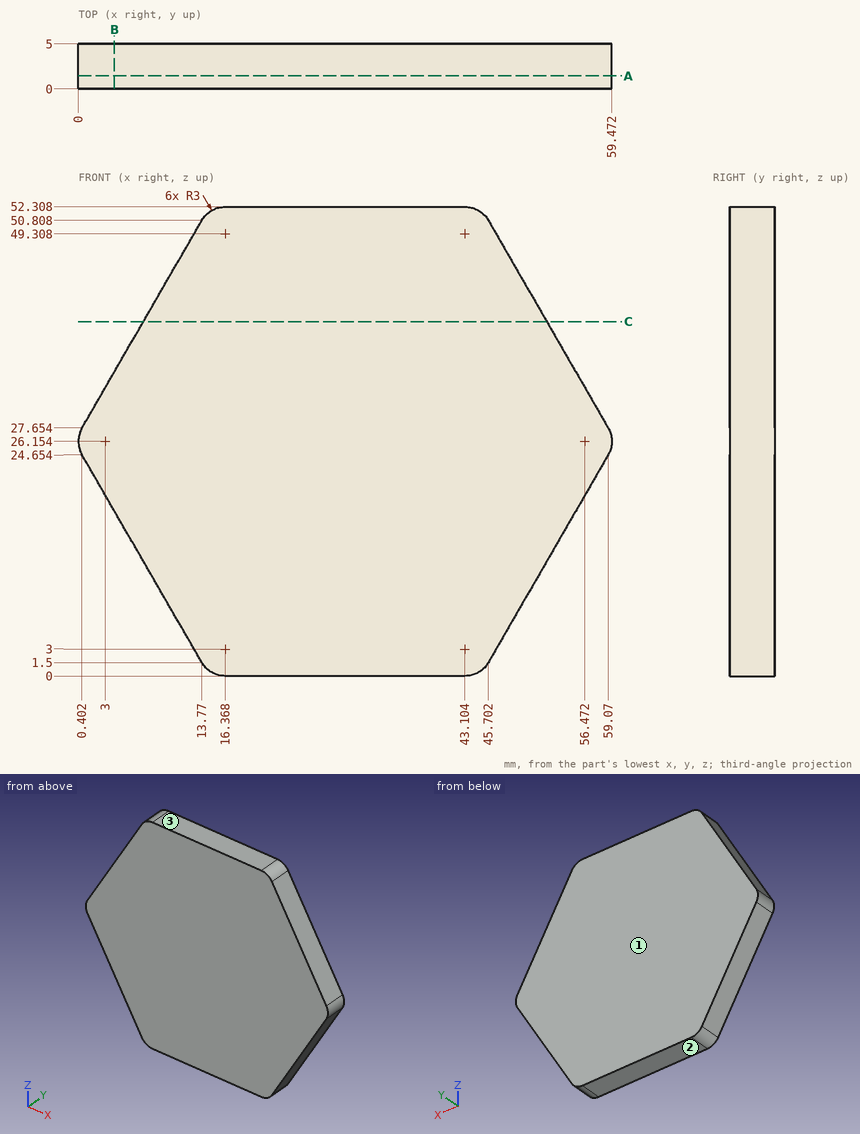
Design review of the part shown in the three views and the two pictorial views. Dimensions are in mm from the part's minimum x, y and z. Round coordinates to 2 decimals unless told otherwise and drop trailing zeros. Loops run counter-clockwise (first coordinate to the right, second up) from the corner with the lowest first, then second, coordinate; pieces in that order, holes last. Notation, with made-up numbers: M -29,56 L 8,56 A32 cw 8,87 Z; hole C 34,87.25 d4. An arc over 180 degrees is marked long. Put each result on its own line as item: value.
Q1. Consider section C-C, the plane z = 39.5. Give the boundary of the cut face in (x, y), then the cut area to 3 significant figures.
Result set:
outline: M 7.24,0 L 52.23,0 L 52.23,5 L 7.24,5 Z
area: 225 mm²
Q2. For pin 1 (1.5 mm diameter, centred on y = 0.5, z = 15.5, fed in from +X), flat-tipped, find the tip position at first contact; note if it passes through.
Result set:
pin 1: stops at x = 54.22
Q3. To check wall thickness, follow L1, parallel to X at y = 4.5, z = 15.5 (1 decimal); L2, parallel to X at y = 3.95, z = 29.5 (1 decimal); L3, parallel to Z at x = 50, y = 3.95 (1 decimal). State the ranges of each line that lie inside material, in increasing order.
Result set:
L1: x = 5.7 to 53.8
L2: x = 1.5 to 58
L3: z = 8.9 to 43.4
Q4. Mouldability with a two-part tool opening along Z and no side actions: class the marked faces 1, 2 and 3 as released by +Z, released by -Z, zero draft, split by the parting line, or undercut.
Result set:
face 1: zero draft
face 2: released by -Z
face 3: released by +Z
Q5. Consider section A-A, the plane y = 1.45. Give the boundary of the cut face in (x, z), then the cut area to 3 significant figures.
Result set:
outline: M 0.4,24.65 L 13.77,1.5 A3 ccw 16.37,0 L 43.1,0 A3 ccw 45.7,1.5 L 59.07,24.65 A3 ccw 59.07,27.65 L 45.7,50.81 A3 ccw 43.1,52.31 L 16.37,52.31 A3 ccw 13.77,50.81 L 0.4,27.65 A3 ccw Z
area: 2,370 mm²
Q6. Consider section B-B, the plane x = 4. Give the boundary of the cut face in (y, z).
Result set:
outline: M 0,18.42 L 5,18.42 L 5,33.89 L 0,33.89 Z
